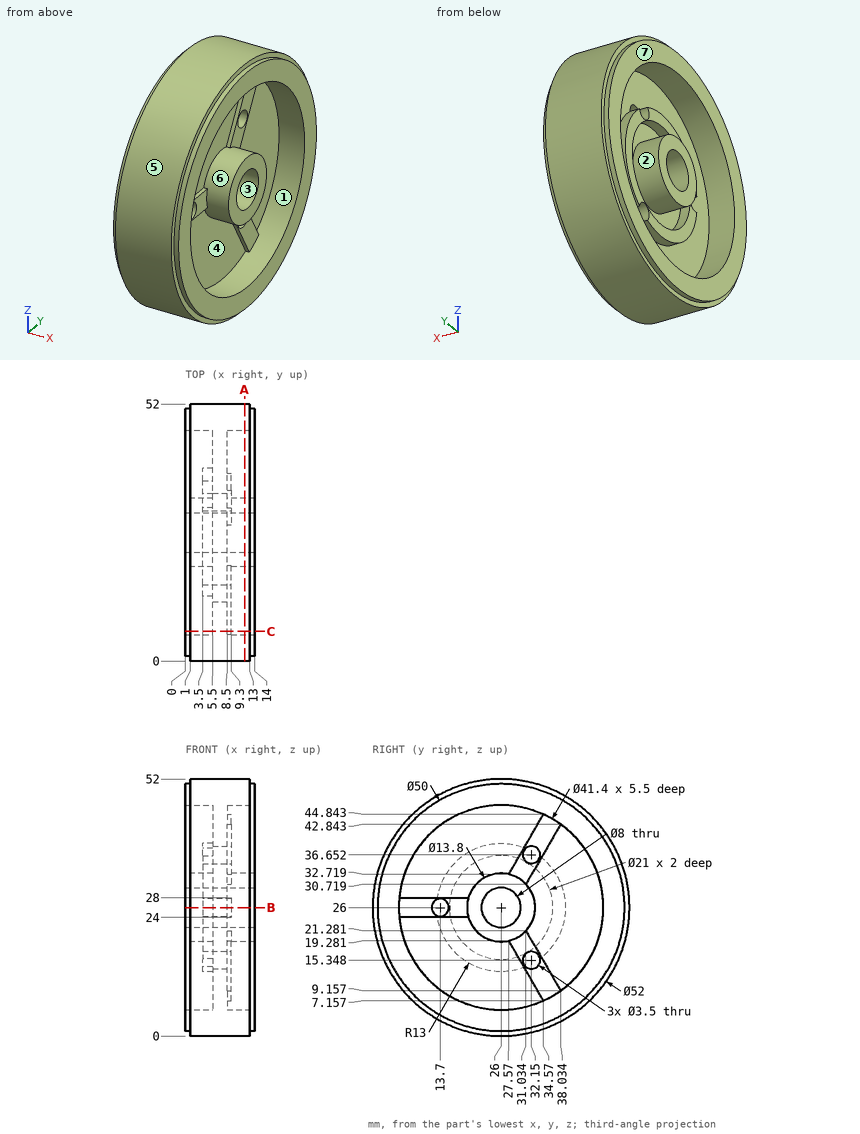
The figure shows three views and two pictorial views of one solid part (mm, origin at its lowest corner). Answer the questions. A direction names the side the tool comes from. Give positions to 0.01 mm unless a question says otherwise; leave off trailing zeros. Write each loop counter-clockwise with the first axis right and the second up, starting at its lowest first coordinate (ties: lowest second). Pieces come first, ordered by that corner, then holes. Notation, with made-up numbers: M -0.75,63 L 31.25,63 A36 ccw 31.25,102 Z; hole C 9,61.25 d10. An arc over 180 degrees is marked long. One line per item, written item: value. Start each with the question number.
(1) Find the intervals of material crossed by line 1 (Y direction, x = 3.45, z = 26); line 2 (Z direction, x = 6.25, y = 32.15), in increasing order.
(2) Determine the mould class of the marked faces 4, 5, 6 and 7 for opening direction Z: pulls with the +Z half, pulls with the -Z half, needs draft (parallel to the pull), parting line crosses it, or undercut.
(3) A tool of negligible diameter and unlimited length cuts with its end or side. For the marked faces 1, 2 and 3, from which of +Z, -Z, +X, -X, +Y, -Y can it reach the whole face along a straight path? Write none if from no direction.
(4) Find section C-C (y = 6). Determine the outline of the cut face in (x, z).
(5) Find section A-A (x = 12). Determine the outline of the cut face in (y, z).
(6) Find section B-B (z = 26). Give the number of separate pieces and of enclosed holes in the cut face, plus the area to 3 significant figures.
(7) Flat-ended cylindrical pins translate along their axes: pin 1 Ø1.5 at (y, z) = (28, 39) entering from +X; pin 2 Ø8 at (y, z) = (26, 9.5) entering from -X; pin 3 Ø1 at (x, y) = (3.5, 45) entering from +Z; pin 4 Ø6.5 at (y, z) = (26, 26) entering from -X. Find the tip coordinate at first contact, or state that the pin passes through.
Results below:
1. line 1: y = 0 to 5.3, 19.1 to 22, 30 to 32.9, 46.7 to 52
1. line 2: z = 0.74 to 13.6, 17.1 to 34.9, 38.4 to 51.26
2. face 4: undercut
2. face 5: parting line crosses it
2. face 6: undercut
2. face 7: needs draft
3. face 1: +X
3. face 2: -X
3. face 3: +X, -X
4. outline: M 0,11 L 1,11 L 1,9.39 L 13,9.39 L 13,11 L 14,11 L 14,20.66 L 8.5,20.66 L 8.5,24 L 9.3,24 L 9.3,28 L 8.5,28 L 8.5,31.34 L 14,31.34 L 14,41 L 13,41 L 13,42.61 L 1,42.61 L 1,41 L 0,41 L 0,31.34 L 5.5,31.34 L 5.5,20.66 L 0,20.66 Z
5. outline: C 26,26 d52; C 26,26 d13.8; hole C 26,26 d41.4; hole C 26,26 d8
6. separate pieces: 3
6. enclosed holes: 0
6. area: 311 mm^2
7. pin 1: stops at x = 8.5
7. pin 2: stops at x = 3.5
7. pin 3: stops at z = 44.27
7. pin 4: passes through
